Autodesk Inventor part; units mm, degrees
ref_plane "YZ Plane" through (0, 0, 0) normal (1, 0, 0) x (0, 1, 0)
ref_plane "XZ Plane" through (0, 0, 0) normal (0, 1, 0) x (-1, 0, 0)
ref_plane "XY Plane" through (0, 0, 0) normal (0, 0, 1) x (1, 0, 0)
sketch "Sketch1" plane through (0, 0, 0) normal (0, 1, 0) x (-1, 0, 0)
  circle A0 centre (0, 0) radius 19
  dimension "d0" = 38
extrude "Extrusion1" add sketch "Sketch1" along normal blind 5
sketch "Sketch2" plane through (0, 5, 0) normal (0, 1, 0) x (1, 0, 0)
  circle A0 centre (-4.5, 0) radius 1.5
  circle A1 centre (4.5, 0) radius 1.5
  point P0 (0, 0)
  dimension "d5" = 3
  dimension "d6" = 3
extrude "Extrusion2" cut sketch "Sketch2" against normal blind 5 contours A0
extrude "Extrusion3" cut sketch "Sketch2" against normal blind 5 contours A1
thread "Thread1"
thread "Thread2"
properties part number "tapa"
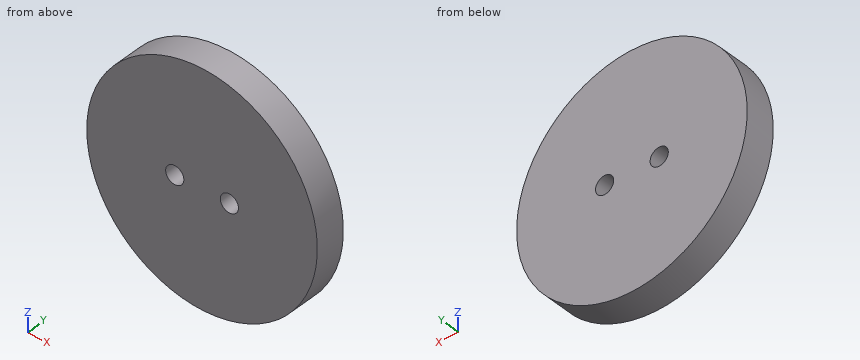
Part model, mm, in its own coordinate system. Round coordinates to 2 decimals unless told otherwise and drop trailing zeros. Loops run counter-clockwise (first coordinate to the right, second up) from the corner with the lowest first, then second, coordinate; pieces in that order, holes last. Notation, with made-up numbers: (15, 68.25) -> (47, 68.25) arc R17 ccw to (47, 78.25) -> close; hole circle Ø5 at (71, 10.25). An arc over 180 degrees is marked (long way). Use CSV: the item, a comma, the result in double quotes. Start each with the question number.
1) Drop flat-ended pins along their axis: P1, Ø1.5, axis at x = 9.5, y = 3, coming from the +Z side; P2, Ø2, axis at y = 3, z = -10, coming from the +X side; P3, Ø1, axis at y = 3.5, z = 2.5, coming from the -X side. Give the stop position or say it passes through.
2) Cut at D-D, the plane z = -11.5. Write the cut outline in (x, y).
3) Cut at B-B, the plane x = 4.5. Write the cut outline in (y, z), plus the area to 3 significant figures.
4) Cut at C-C, the plane y = 3.7. Write the cut outline in (x, z), plus the area to 3 significant figures.
5) Cut at A-A, the plane z = 0. Write the cut outline in (x, y), plus the area to 3 significant figures.
6) Wall check: L1, parallel to Z at x = -5, y = 4.3; L2, parallel to Z at x = 4.5, y = 1.35; L3, parallel to X at y = 4, z = -3. Give the ranges that are in metal, low to high. Write a range as [from, to].
Determined:
1,P1,"stops at z = 16.87"
1,P2,"stops at x = 16.73"
1,P3,"stops at x = -18.89"
2,outline,"(-15.12, 0) -> (15.12, 0) -> (15.12, 5) -> (-15.12, 5) -> close"
3,outline,"(0, -18.46) -> (5, -18.46) -> (5, -1.5) -> (0, -1.5) -> close; (0, 1.5) -> (5, 1.5) -> (5, 18.46) -> (0, 18.46) -> close"
3,area,"170 mm2"
4,outline,"circle Ø38 at (0, 0); hole circle Ø3 at (-4.5, 0); hole circle Ø3 at (4.5, 0)"
4,area,"1,120 mm2"
5,outline,"(-19, 0) -> (-6, 0) -> (-6, 5) -> (-19, 5) -> close; (-3, 0) -> (3, 0) -> (3, 5) -> (-3, 5) -> close; (6, 0) -> (19, 0) -> (19, 5) -> (6, 5) -> close"
5,area,"160 mm2"
6,L1,"z = [-18.33, -1.41], [1.41, 18.33]"
6,L2,"z = [-18.46, -1.5], [1.5, 18.46]"
6,L3,"x = [-18.76, 18.76]"
